Verification items for the finished model (mm, model axes). Face numbers are marked on the shaded views. A direction names the side the tool comes from. Coordinates: 2 decimals unless noted, no trailing zeros. Write each loop counter-clockwise with the first axis right and the second up, starting at its lowest first coordinate (ties: lowest second). Pieces come first, ordered by that corner, then holes. Notation, with made-up numbers: (37.25, 85.5) - (95.25, 85.5) arc R32 cw to (95.25, 116.5) - close; hole circle Ø5 at (11, -27). An arc over 180 degrees is marked (long way). Answer as CSV lines item,"result". Start each with the question number.
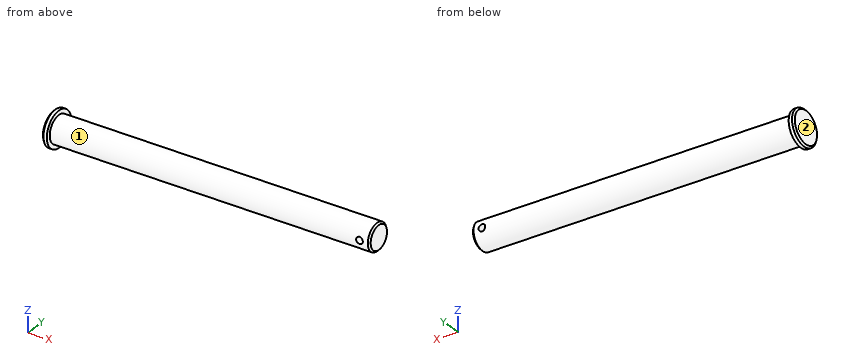
```python
from build123d import *

# Parameters (mm, degrees)
SZKIC2_R                        = 2
WYTNIJ_WYCI_GNI_CIE1_DEPTH      = 11.5
WYTNIJ_WYCI_GNI_CIE1_DEPTH_BACK = 11.5
SFAZOWANIE1_SIZE                = 1


with BuildPart() as part:
    # Szkic1 → Obrót1 (revolve)
    with BuildSketch(Plane.XY):
        Polygon((0, 0), (0, 10.5), (3, 10.5), (3, 8), (194, 8), (194, 0), align=None)
    revolve(axis=Axis((194, 0, 0), (-1, 0, 0)))

    # Szkic2 → Wytnij-wyciągnięcie1 (cut, two sides)
    with BuildSketch(Plane(origin=(0, 0, 0), x_dir=(1, 0, 0), z_dir=(0, 1, 0))) as wytnij_wyci_gni_cie1_sk:
        with Locations((188, 0)):
            Circle(SZKIC2_R)
    extrude(amount=WYTNIJ_WYCI_GNI_CIE1_DEPTH, mode=Mode.SUBTRACT)
    extrude(wytnij_wyci_gni_cie1_sk.sketch, amount=-WYTNIJ_WYCI_GNI_CIE1_DEPTH_BACK, mode=Mode.SUBTRACT)

    # Sfazowanie1
    sfazowanie1_edges = [part.edges().sort_by_distance(p)[0] for p in [
        (194, -8, 0),
        (0, -10.5, 0),
    ]]
    chamfer(sfazowanie1_edges, length=SFAZOWANIE1_SIZE)


solid = part.part
```
1. Access from +Z, -Z, +X, -X, +Y, -Y to the whole of each face (thin tool, end or side, straight path). Record for the marked faces 1 and 2.
2. Cross-section at B-B (x = 134.5). Record the cut outline in (y, z), and give its area (3 significant figures).
3. Scan lines: line 1 along X through (y, z) = (-1.5, 0); line 2 along X through (y, z) = (-3, 1.5); line 3 along X through (y, z) = (-5.25, -7). Record each from-to range of solid material in increasing order. Write a range as from..to.
4. Depth check by flat-ended pin: P1, Ø12, axis at x = 152.5, y = 5, coming from the -Z side; P2, Ø5, axis at x = 188, z = 0, coming from the -Y side; P3, Ø8, axis at x = 152, y = -7, coming from the -Z side; P4, Ø3, axis at x = 188, z = 0, coming from the -Y side. Enter the tip coordinate at first touch or a pass-through.
5. Cross-section at A-A (x = 188). Record the cut outline in (y, z).
Completed:
1,face 1,"+X"
1,face 2,"+Z, -Z, -X, +Y, -Y"
2,outline,"circle Ø16 at (0, 0)"
2,area,"201 mm2"
3,line 1,"x = 0..186, 190..194"
3,line 2,"x = 0..186.68, 189.32..194"
3,line 3,"x = 0..3"
4,P1,"stops at z = -8"
4,P2,"stops at y = -8"
4,P3,"stops at z = -7.42"
4,P4,"passes through"
5,outline,"(-7.75, -2) arc R8 ccw to (7.75, -2) - close; (-7.75, 2) - (7.75, 2) arc R8 ccw to start"
